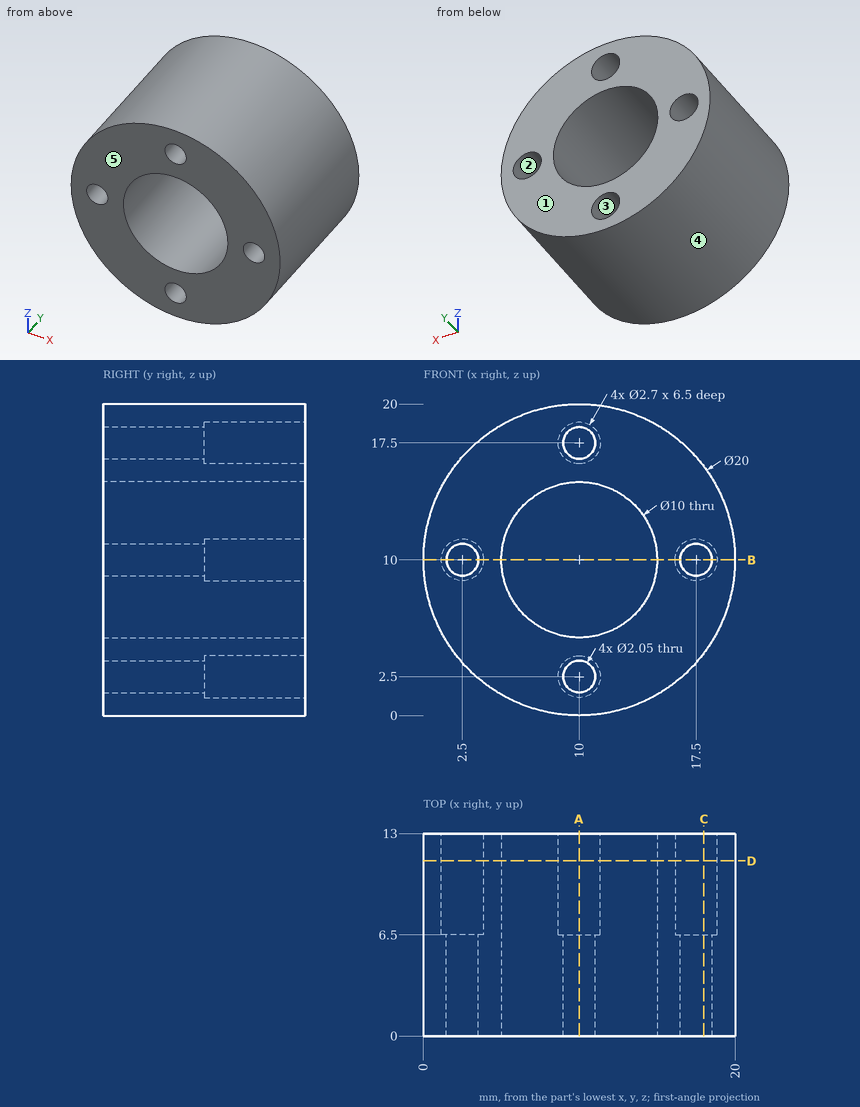
Geometry: see drawing. Coordinates: mm, zero at the bounding-box minimum. A direction names the side the tool comes from. Give positions to 0.01 mm unless a question says otherwise; leave off trailing zeros. Write each loop counter-clockwise with the first axis right and the second up, starting at its lowest first coordinate (ties: lowest second). Pieces come first, ordered by that corner, then holes. Notation, with made-up numbers: (-28.75, 46.5) -> (-5.75, 46.5) arc R18 cw to (-5.75, 76.5) -> close; hole circle Ø3 at (11.25, 15.5). An arc over 180 degrees is marked (long way). Use one line per item in the form item = value. Start each with the question number.
1) Section query B-B on z = 10. Return the cut outline in (x, y) (3 decimals).
2) Section query A-A on x = 10. Return the cut outline in (y, z) (3 decimals).
3) Draft query along X for the marked faces 3, 4 and 5. Return one class per face: pulls with the +X half, pulls with the -X half, needs draft (parallel to the pull), parting line crosses it, or undercut.
4) Section query C-C on x = 18. Return the cut outline in (y, z), then the cut area to 3 significant figures.
5) Ray query, probe 1 along X at (y, z) = (8.75, 2.5); probe 2 along Z at (x, y) = (13, 6); probe 3 along X at (y, z) = (2.75, 2.5) (3 decimals). Return the intervals inside material, ascending. Write a range as from..to.
6) Section query D-D on y = 11.25. Return the cut outline in (x, z).
7) Pin query (flat end, axial travel): pin 1 (2 mm diameter, centred on x = 18, y = 3.5, fed in from +Z); pin 2 (1 mm diameter, centred on x = 15.5, y = 4, fed in from -Z); pin 3 (1 mm diameter, centred on x = 7, y = 9.5, fed in from -Z). Return the tip coordinate at first contact, or that it passes through.
8) Set-up query: the marked faces 1 and 2. Return all of +Z, -Z, +X, -X, +Y, -Y with unobstructed straight access to the full face (end or side cutting, diameter ignored); none if empty.
Outcome:
q1.outline = (0, 0) -> (1.475, 0) -> (1.475, 6.5) -> (1.15, 6.5) -> (1.15, 13) -> (0, 13) -> close; (3.525, 0) -> (5, 0) -> (5, 13) -> (3.85, 13) -> (3.85, 6.5) -> (3.525, 6.5) -> close; (15, 0) -> (16.475, 0) -> (16.475, 6.5) -> (16.15, 6.5) -> (16.15, 13) -> (15, 13) -> close; (18.525, 0) -> (20, 0) -> (20, 13) -> (18.85, 13) -> (18.85, 6.5) -> (18.525, 6.5) -> close
q2.outline = (0, 0) -> (13, 0) -> (13, 1.15) -> (6.5, 1.15) -> (6.5, 1.475) -> (0, 1.475) -> close; (0, 3.525) -> (6.5, 3.525) -> (6.5, 3.85) -> (13, 3.85) -> (13, 5) -> (0, 5) -> close; (0, 15) -> (13, 15) -> (13, 16.15) -> (6.5, 16.15) -> (6.5, 16.475) -> (0, 16.475) -> close; (0, 18.525) -> (6.5, 18.525) -> (6.5, 18.85) -> (13, 18.85) -> (13, 20) -> (0, 20) -> close
q3.face_3 = undercut
q3.face_4 = parting line crosses it
q3.face_5 = needs draft
q4.outline = (0, 4) -> (13, 4) -> (13, 8.75) -> (6.5, 8.75) -> (6.5, 9.11) -> (0, 9.11) -> close; (0, 10.89) -> (6.5, 10.89) -> (6.5, 11.25) -> (13, 11.25) -> (13, 16) -> (0, 16) -> close
q4.area = 128 mm^2
q5.probe_1 = 3.39..8.65, 11.35..16.61
q5.probe_2 = 0.46..6, 14..19.54
q5.probe_3 = 3.386..8.975, 11.025..16.614
q6.outline = circle Ø20 at (10, 10); hole circle Ø2.7 at (2.5, 10); hole circle Ø10 at (10, 10); hole circle Ø2.7 at (10, 2.5); hole circle Ø2.7 at (10, 17.5); hole circle Ø2.7 at (17.5, 10)
q7.pin_1 = 17.14
q7.pin_2 = 1.34
q7.pin_3 = 0.32
q8.face_1 = +Z, -Z, +X, -X, +Y
q8.face_2 = +Y
